Source: three-view drawing plus pictorial views. Frame: mm from the lowest corner of the part. A direction names the side the tool comes from. Coordinates: 2 decimals unless noted, no trailing zeros. Loops run counter-clockwise (first coordinate to the right, second up) from the corner with the lowest first, then second, coordinate; pieces in that order, holes last. Notation, with made-up numbers: (3.25, 33) - (9.25, 33) arc R29 cw to (9.25, 59) - close; hole circle Ø5 at (89, 48.5). An arc over 180 degrees is marked (long way). Return JSON: item names as keys, results as strings.
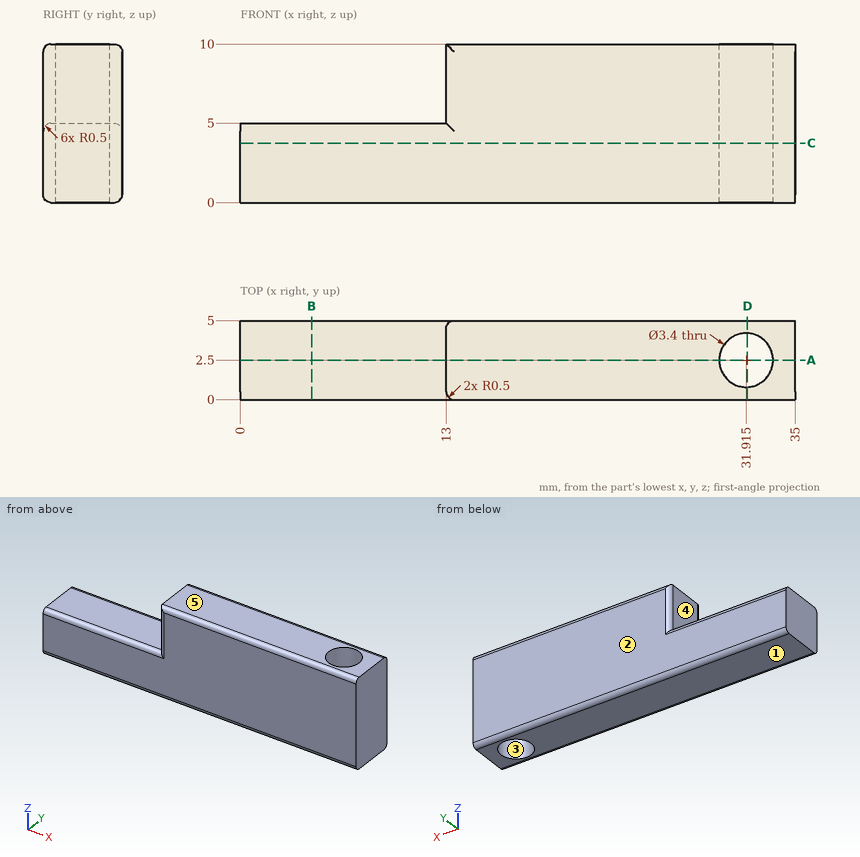
Item 1: Mould query, pull axis Y, two halves, no side actions, for the marked faces 1, 2 and 3. Classes: +Y half, -Y half, draft (parallel to the pull), parting line (faces both ways), or undercut.
Worked out:
{"face 1": "draft", "face 2": "+Y half", "face 3": "undercut"}
Item 2: Ray query, probe 1 along X at (y, z) = (2.65, 1.25); probe 2 along X at (y, z) = (2.4, 6.5); probe 3 along Z at (x, y) = (12, 3.15). Return the intervals inside material, ascending. Write a range as from..to.
Worked out:
{"probe 1": "0..30.22, 33.61..35", "probe 2": "13..30.22, 33.61..35", "probe 3": "0..5"}
Item 3: Section query A-A, the plane y = 2.5. Return loops of the section in (x, z) (1 decimal).
Worked out:
{"outline": "(0, 0) - (30.2, 0) - (30.2, 10) - (13, 10) - (13, 5) - (0, 5) - close; (33.6, 0) - (35, 0) - (35, 10) - (33.6, 10) - close"}
Item 4: Section query C-C, the plane z = 3.75. Return loops of the section in (x, y) (1 decimal), and give its area (3 significant figures).
Worked out:
{"outline": "(0, 0) - (35, 0) - (35, 5) - (0, 5) - close; hole circle Ø3.4 at (31.9, 2.5)", "area": "166 mm^2"}
Item 5: Section query D-D, the plane x = 32. Return loops of the section in (y, z).
Worked out:
{"outline": "(0, 0.5) arc R0.5 ccw to (0.5, 0) - (0.8, 0) - (0.8, 10) - (0.5, 10) arc R0.5 ccw to (0, 9.5) - close; (4.2, 0) - (4.5, 0) arc R0.5 ccw to (5, 0.5) - (5, 9.5) arc R0.5 ccw to (4.5, 10) - (4.2, 10) - close"}
Item 6: Reachability of the marked faces 4 and 5 from +Z, -Z, +X, -X, +Y, -Y: full face, straight path, thin tool, end or side. Return the list, or none.
Worked out:
{"face 4": "+Z, -X, +Y, -Y", "face 5": "+Z, +X, -X, +Y, -Y"}
Item 7: Section query B-B, the plane x = 4.5. Return loops of the section in (y, z), and give its area (3 significant figures).
Worked out:
{"outline": "(0, 0.5) arc R0.5 ccw to (0.5, 0) - (4.5, 0) arc R0.5 ccw to (5, 0.5) - (5, 4.5) arc R0.5 ccw to (4.5, 5) - (0.5, 5) arc R0.5 ccw to (0, 4.5) - close", "area": "24.8 mm^2"}
Item 8: First-contact query: pin 1 Ø1 at (x, z) = (24.5, 8.5) entering from -Y; pin 2 Ø3 at (x, y) = (5, 2.5) entering from +Z; pin 3 Ø1.2 at (y, z) = (3.5, 8) entering from -X. Flat tips, straight axial feed; report the tip coordinate or a pass-through.
Worked out:
{"pin 1": "y = 0", "pin 2": "z = 5", "pin 3": "x = 13"}
